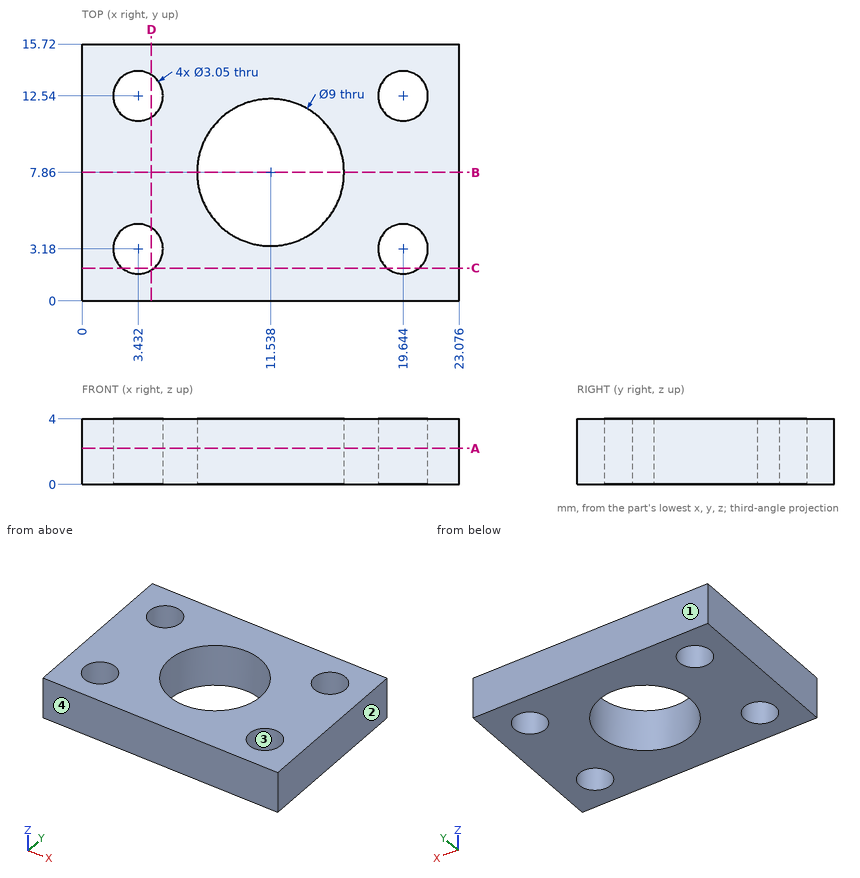
Can you work these out from the drawing? Everything is in mm from the part's minimum corner. Round coordinates to 2 decimals unless told otherwise and drop trailing zeros. Order: outer loops, then holes, each group sorted by start corner. A loop starts at its lowest first (then second) coordinate and runs counter-clockwise, first axis right, second up. Notation, with made-up numbers: (72.25, 81.5) -> (82.25, 81.5) arc R16 cw to (82.25, 107.5) -> close; hole circle Ø5 at (-13.5, 19). An arc over 180 degrees is marked (long way). Use CSV: the item, a comma, the result in double quotes.
1. I want a section at D-D on x = 4.25. List the corners of the cut face in (y, z) for me, and give its area (3 significant figures).
Recorded:
outline,"(0, 0) -> (1.89, 0) -> (1.89, 4) -> (0, 4) -> close; (4.47, 0) -> (11.25, 0) -> (11.25, 4) -> (4.47, 4) -> close; (13.83, 0) -> (15.72, 0) -> (15.72, 4) -> (13.83, 4) -> close"
area,"42.3 mm2"
2. I want a section at A-A on z = 2.2. List the corners of the cut face in (x, y) for me (3 decimals), and give its area (3 significant figures).
Recorded:
outline,"(0, 0) -> (23.076, 0) -> (23.076, 15.72) -> (0, 15.72) -> close; hole circle Ø3.05 at (3.432, 3.18); hole circle Ø3.05 at (3.432, 12.54); hole circle Ø9 at (11.538, 7.86); hole circle Ø3.05 at (19.644, 3.18); hole circle Ø3.05 at (19.644, 12.54)"
area,"270 mm2"
3. I'm going to push a flat-ended pin straight in: P1, Ø2, axis at x = 19, z = 2, coming from the -Y side. Where does the tip first touch, or does it pass through?
Recorded:
P1,"stops at y = 0"
4. I want a section at C-C on y = 2. List the corners of the cut face in (x, z) for me.
Recorded:
outline,"(0, 0) -> (2.47, 0) -> (2.47, 4) -> (0, 4) -> close; (4.4, 0) -> (18.68, 0) -> (18.68, 4) -> (4.4, 4) -> close; (20.61, 0) -> (23.08, 0) -> (23.08, 4) -> (20.61, 4) -> close"
5. I need wall thicknesses on line 1 along X through (y, z) = (2.75, 2) (3 decimals); line 2 along X through (y, z) = (13.5, 1.05); line 3 along Y through (x, z) = (4.5, 2.2). Which ranges of each line are inside material? Lowest first, please.
Recorded:
line 1,"x = 0 to 1.969, 4.895 to 18.181, 21.107 to 23.076"
line 2,"x = 0 to 2.25, 4.62 to 18.46, 20.83 to 23.08"
line 3,"y = 0 to 2.09, 4.27 to 11.45, 13.63 to 15.72"
6. Thinking about a two-plate mould opening in Y: for the marked faces 1, 2, 3 and 4, which applies, pulls with the +Y half, pulls with the -Y half, needs draft (parallel to the pull), parting line crosses it, or undercut?
Recorded:
face 1,"pulls with the +Y half"
face 2,"needs draft"
face 3,"undercut"
face 4,"pulls with the -Y half"
7. I want a section at B-B on y = 7.86. List the corners of the cut face in (x, z) for me.
Recorded:
outline,"(0, 0) -> (7.04, 0) -> (7.04, 4) -> (0, 4) -> close; (16.04, 0) -> (23.08, 0) -> (23.08, 4) -> (16.04, 4) -> close"
